from build123d import *

# Parameters (mm, degrees)
BOSS_EXTRUDE1_DEPTH = 225
SKETCH2_R           = 4.5
CUT_EXTRUDE5_DEPTH  = 101
SKETCH6_R           = 8
CUT_EXTRUDE6_DEPTH  = 98


with BuildPart() as part:
    # Sketch1 → Boss-Extrude1 (new body)
    with BuildSketch(Plane.XY):
        Polygon((-60, -52.594339623), (0, -52.594339623), (0, 47.405660377), (-29.586723225, 15.796476851), align=None)
    extrude(amount=BOSS_EXTRUDE1_DEPTH)

    # Sketch2 → Cut-Extrude5 (cut, through all)
    with BuildSketch(Plane.XZ.offset(52.594339623)):
        with Locations((-30, 202.5)):
            Circle(SKETCH2_R)
        with Locations((-30, 22.5)):
            Circle(SKETCH2_R)
    extrude(amount=-CUT_EXTRUDE5_DEPTH, mode=Mode.SUBTRACT)

    # Sketch6 → Cut-Extrude6 (cut, through all)
    with BuildSketch(Plane(origin=(0, -49.594339623, 0), x_dir=(-1, 0, 0), z_dir=(0, -1, 0))):
        with Locations((30, -22.5)):
            Circle(SKETCH6_R)
        with Locations((30, -202.5)):
            Circle(SKETCH6_R)
    extrude(amount=-CUT_EXTRUDE6_DEPTH, mode=Mode.SUBTRACT)


solid = part.part
Geometry check sheet. Reference: the model listing, model coordinates, mm. A direction names the side the tool comes from. Give positions to 0.01 mm unless a question says otherwise; leave off trailing zeros. Loops run counter-clockwise (first coordinate to the right, second up) from the corner with the lowest first, then second, coordinate; pieces in that order, holes last. Notation, with made-up numbers: (-11, 81.25) -> (13, 81.25) arc R21 ccw to (13, 112.25) -> close; hole circle Ø3 at (34.5, -6.75). An arc over 180 degrees is marked (long way). Answer in a Markdown table with one row per item. Add a question column.
1) Cross-section at A-A on z = 22.5. Record the boundary of the cut face in (x, y), and give its area (3 significant figures).
2) Cross-section at C-C on y = 2. Record the boundary of the cut face in (x, z).
3) Cross-section at B-B on y = -41.5. Record the boundary of the cut face in (x, z).
4) Gauge pin test, flat ends, axial feed: P1, Ø14.5, axis at x = -30, z = 202.5, coming from the +Y side; P2, Ø1, axis at x = -7, z = 134, coming from the +Y side; P3, Ø2, axis at x = -18, z = 41.5, coming from the +Y side. Record the tip position at first contact, or that the pin passes through.
5) Set-up check for faces 5 (the face through (-30.98, -51.12, 198.11)), 6 (the face through (-22.008, -21.42, 22.148)): record each of +Z, -Z, +X, -X, +Y, -Y from which the full face is reachable in a straight line by a thin tool's end or side.
6) Cross-section at D-D on z = 93. Record the boundary of the cut face in (x, y), and give its area (3 significant figures).
7) Material ranges on probe 1 along Z at (x, y) = (-30, -24); probe 2 along X at (y, z) = (6, 202.5); probe 3 along X at (y, z) = (-15, 202), recorded low to high. Write a range as from..to.
8) Draft check along X on faces 1 (the face through (-14.59, 31.82, 110.92)), 2 (the face through (0, -3, 111)), 3 (the face through (-33.4, -49.594, 25.9)), 4 (the face through (-24, -13, 0)). Enter one of: pulls with the +X half, pulls with the -X half, needs draft (parallel to the pull), parting line crosses it, or undercut.
Outcome:
| question | item | result |
|---|---|---|
| 1 | outline | (-60, -52.59) -> (-34.5, -52.59) -> (-34.5, -49.59) -> (-38, -49.59) -> (-38, -3.12) -> close; (-25.5, -52.59) -> (0, -52.59) -> (0, 47.41) -> (-22, 23.9) -> (-22, -49.59) -> (-25.5, -49.59) -> close |
| 1 | area | 2,510 mm^2 |
| 2 | outline | (-35.72, 0) -> (0, 0) -> (0, 225) -> (-35.72, 225) -> (-35.72, 208.09) arc R8 cw (long way) to (-35.72, 196.91) -> (-35.72, 28.09) arc R8 cw (long way) to (-35.72, 16.91) -> close |
| 3 | outline | (-55.07, 0) -> (0, 0) -> (0, 225) -> (-55.07, 225) -> close; hole circle Ø16 at (-30, 22.5); hole circle Ø16 at (-30, 202.5) |
| 4 | P1 | stops at y = -49.59 |
| 4 | P2 | stops at y = 40.46 |
| 4 | P3 | stops at y = 29.24 |
| 5 | face 5 | +Y, -Y |
| 5 | face 6 | +Y |
| 6 | outline | (-60, -52.59) -> (0, -52.59) -> (0, 47.41) -> (-29.59, 15.8) -> close |
| 6 | area | 3,530 mm^2 |
| 7 | probe 1 | z = 0..14.5, 30.5..194.5, 210.5..225 |
| 7 | probe 2 | x = -22..0 |
| 7 | probe 3 | x = -43.28..-37.98, -22.02..0 |
| 8 | face 1 | pulls with the -X half |
| 8 | face 2 | pulls with the +X half |
| 8 | face 3 | undercut |
| 8 | face 4 | needs draft |
